```python
from build123d import *

# Parameters (mm, degrees)
SKETCH_1_W          = 33
SKETCH_1_H          = 18
SKETCH_2_W          = 14
SKETCH_2_H          = 3
SKETCH_2_W_2        = 2.671402587
SKETCH_2_H_2        = 6
CUT_EXTRUDE_START   = -30
SKETCH_4_R          = 1.5
CUT_EXTRUDE_1_DEPTH = 1


with BuildPart() as part:
    # 草图1 → 旋转1 (revolve)
    with BuildSketch(Plane.XY, mode=Mode.PRIVATE) as revolve_1_sk:
        Polygon((0, 18.5), (0, 18), (0, 0), (-30, 0), (-30, 18.5), align=None)
        with Locations((16.5, 9)):
            Rectangle(SKETCH_1_W, SKETCH_1_H)
        with BuildLine():
            Line((33, 5), (33, 0))
            Line((33, 0), (36, 0))
            Line((36, 0), (36, 4))
            ThreePointArc((36, 4), (35.707106781, 4.707106781), (35, 5))
            Line((35, 5), (33, 5))
        make_face()
    revolve(revolve_1_sk.sketch.rotate(Axis((-39.714285714, 0, 0), (1, 0, 0)), 90), axis=Axis((-39.714285714, 0, 0), (1, 0, 0)))

    # 草图2 → 旋转3 (revolve)
    with BuildSketch(Plane.XY, mode=Mode.PRIVATE) as revolve_3_sk:
        with Locations((-39.671402587, 10.75)):
            Rectangle(SKETCH_2_W, SKETCH_2_H)
        with Locations((-31.335701294, 12.25)):
            Rectangle(SKETCH_2_W_2, SKETCH_2_H_2)
    revolve(revolve_3_sk.sketch.rotate(Axis((-54.775263054, 9.25, 0), (1, 0, 0)), 180), axis=Axis((-54.775263054, 9.25, 0), (1, 0, 0)))

    # 草图4 → 切除-拉伸1 (cut)
    with BuildSketch(Plane(origin=(0, 0, 0), x_dir=(0, 0, -1), z_dir=(1, 0, 0)).offset(CUT_EXTRUDE_START)):
        with Locations((8, 0.25)):
            Circle(SKETCH_4_R)
        with Locations((-8, 0.25)):
            Circle(SKETCH_4_R)
    extrude(amount=CUT_EXTRUDE_1_DEPTH, mode=Mode.SUBTRACT)


solid = part.part
```
Geometry: final body of the model. Coordinates: model frame, mm. A direction names the side the tool comes from. Round coordinates to 2 decimals unless told otherwise and drop trailing zeros. Loops run counter-clockwise (first coordinate to the right, second up) from the corner with the lowest first, then second, coordinate; pieces in that order, holes last. Notation, with made-up numbers: (-40, -10) -> (-3, -10) arc R26 ccw to (-3, 11) -> close; hole circle Ø6 at (64, 53). An arc over 180 degrees is marked (long way). Use one line per item in the form item = value. Start each with the question number.
1) Section D-D on z = -8. Output: boundary loops of the cut face in (x, y), then the cut area to 3 significant figures.
2) Section B-B on y = 7.5. Output: boundary loops of the cut face in (x, z).
3) Draft query along Z for faces 4 (the cylindrical face through (16.731, -12.165, -13.267)), 5 (the flat face through (-29, 0, 8)), 6 (the flat face through (-46.671, 9, 0)). Return one class per face: released by +Z, released by -Z, zero draft, split by the parting line, or undercut.
4) Line query: L1, parallel to X at y = -10, z = 8; L2, parallel to Y at x = -29.75, z = -8; L3, parallel to X at y = 5.5, z = -4. Output: solid intervals per line, ascending.
5) First-contact query: P1, Ø10, axis at y = 0.5, z = -13, coming from the +X side; P2, Ø2, axis at y = -9, z = -2, coming from the -X side; P3, Ø1.5, axis at x = -21, z = -9.5, coming from the -Y side. Flat tips, straight axial feed; report the tip coordinate or a pass-through.
6) Section C-C on z = 16. Output: boundary loops of the cut face in (x, y), then the cut area to 3 significant figures.
7) Access query for faces 1 (the cylindrical face through (-31.317, 3.527, -1.802)), 2 (the cylindrical face through (-14.79, 16.41, 8.54)), 3 (the flat face through (33, 4, -4)). Directions: +Z, -Z, +X, -X, +Y, -Y. A direction counts if a zero-diameter tool reaches every point of the face in a straight line with its end or side. Return the directions, or none.
8) Section A-A on z = 0. Output: boundary loops of the cut face in (x, y), then the cut area to 3 significant figures.
Response:
q1.outline = (-30, -16.68) -> (0, -16.68) -> (0, -16.12) -> (33, -16.12) -> (33, 16.12) -> (0, 16.12) -> (0, 16.68) -> (-30, 16.68) -> (-30, 1.75) -> (-29, 1.75) -> (-29, -1.25) -> (-30, -1.25) -> close
q1.area = 2,060 mm^2
q2.outline = (-46.67, -2.44) -> (-32.67, -2.44) -> (-32.67, -5.74) -> (-30, -5.74) -> (-30, -16.91) -> (0, -16.91) -> (0, -16.36) -> (33, -16.36) -> (33, 16.36) -> (0, 16.36) -> (0, 16.91) -> (-30, 16.91) -> (-30, 5.74) -> (-32.67, 5.74) -> (-32.67, 2.44) -> (-46.67, 2.44) -> close
q3.face_4 = split by the parting line
q3.face_5 = undercut
q3.face_6 = zero draft
q4.L1 = -30 to 33
q4.L2 = -16.68 to -1.25, 1.75 to 16.68
q4.L3 = -32.67 to 33
q5.P1 = 33
q5.P2 = -30
q5.P3 = -16.3
q6.outline = (-30, -9.29) -> (0, -9.29) -> (0, -8.25) -> (33, -8.25) -> (33, 8.25) -> (0, 8.25) -> (0, 9.29) -> (-30, 9.29) -> close
q6.area = 1,100 mm^2
q7.face_1 = -X
q7.face_2 = +X, -X
q7.face_3 = +X
q8.outline = (-46.67, 6.25) -> (-32.67, 6.25) -> (-32.67, 3.25) -> (-30, 3.25) -> (-30, -18.5) -> (0, -18.5) -> (0, -18) -> (33, -18) -> (33, -5) -> (35, -5) arc R1 ccw to (36, -4) -> (36, 4) arc R1 ccw to (35, 5) -> (33, 5) -> (33, 18) -> (0, 18) -> (0, 18.5) -> (-30, 18.5) -> (-30, 15.25) -> (-32.67, 15.25) -> (-32.67, 12.25) -> (-46.67, 12.25) -> close
q8.area = 2,440 mm^2
